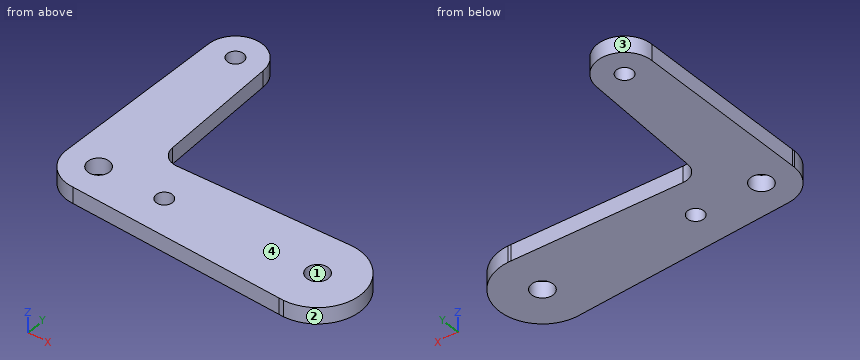
```python
from build123d import *

# Parameters (mm, degrees)
BOSS_EXTRUDE1_DEPTH = 4.7752
FILLET1_R           = 4.7752
SKETCH2_R           = 3.175
SKETCH2_R_2         = 2.3876
CUT_EXTRUDE1_DEPTH  = 4.7752


with BuildPart() as part:
    # Sketch1 → Boss-Extrude1 (new body)
    with BuildSketch(Plane.XY):
        with BuildLine():
            ThreePointArc((7.9502, 50.8), (0, 58.7502), (-7.9502, 50.8))
            Line((-7.9502, 50.8), (-9.506710526, 0.589983026))
            Line((-9.506710526, 0.589983026), (-9.525, 0))
            ThreePointArc((-9.525, 0), (-6.735192091, -6.735192091), (0, -9.525))
            Line((0, -9.525), (62.233167082, -12.636658354))
            Line((62.233167082, -12.636658354), (63.5, -12.7))
            ThreePointArc((63.5, -12.7), (76.2, 0), (63.5, 12.7))
            Line((63.5, 12.7), (62.713355965, 12.675614035))
            Line((62.713355965, 12.675614035), (9.183498158, 11.016188443))
            Line((9.183498158, 11.016188443), (7.9502, 50.8))
        make_face()
        with BuildLine():
            ThreePointArc((9.506710526, 0.589983026), (9.520426534, 0.295133223), (9.525, 0))
            Line((9.525, 0), (9.506710526, 0.589983026))
        make_face(mode=Mode.SUBTRACT)
    extrude(amount=BOSS_EXTRUDE1_DEPTH)

    # Fillet1
    fillet1_edges = [part.edges().sort_by_distance(p)[0] for p in [
        (9.183498158, 11.016188443, 2.3876),
    ]]
    fillet(fillet1_edges, radius=FILLET1_R)

    # Sketch2 → Cut-Extrude1 (cut)
    with BuildSketch(Plane.XY.offset(4.7752)):
        Circle(SKETCH2_R)
        with Locations((0, 50.8)):
            Circle(SKETCH2_R_2)
        with Locations((19.05, 0)):
            Circle(SKETCH2_R_2)
        with Locations((63.5, 0)):
            Circle(SKETCH2_R)
    extrude(amount=-CUT_EXTRUDE1_DEPTH, mode=Mode.SUBTRACT)


solid = part.part
```
Work out the finished part from the listing and answer in its coordinate system (mm). Face numbers are marked on the shaded views. Give positions to 0.01 mm unless a question says otherwise; leave off trailing zeros. Loops run counter-clockwise (first coordinate to the right, second up) from the corner with the lowest first, then second, coordinate; pieces in that order, holes last. Notation, with made-up numbers: (65.25, 45.5) -> (82.25, 45.5) arc R37 cw to (82.25, 84.5) -> close; hole circle Ø5 at (17, -14). An arc over 180 degrees is marked (long way). One line per question, with ' | ' between items. Start each with the question number.
1) Section C-C, the plane y = 18 is taken. Determine the outline of the cut face in (x, z).
2) Section B-B, the plane x = 19.5 is taken. Determine the outline of the cut face in (y, z).
3) Determine the mould class of the marked faces 1, 2, 3 and 4 for opening direction X: +X half, -X half, draft (parallel to the pull), parting line (faces both ways), or undercut.
4) Section A-A, the plane z = 3.3 is taken. Determine the outline of the cut face in (x, y) (3 decimals).
5) This flat-tipped pin is pushed along its axis until it touches: pin 1 (1.5 mm diameter, centred on y = 31, z = 3.5, fed in from -X). Where does it stop, or does it pass through?
6) Straight lines are drawn through the part: L1, parallel to Y at x = 0, z = 2.9 (3 decimals); L2, parallel to Y at x = 63.5, z = 1.85 (3 decimals); L3, parallel to Y at x = 19.5, z = 0.3. For each, find the intervals that lie inside material, in ascending order.
7) Section D-D, the plane x = 55.5 is taken. Determine the outline of the cut face in (y, z), then the cut area to 3 significant figures.
Resolved:
1) outline: (-8.97, 0) -> (8.97, 0) -> (8.97, 4.78) -> (-8.97, 4.78) -> close
2) outline: (-10.5, 0) -> (-2.34, 0) -> (-2.34, 4.78) -> (-10.5, 4.78) -> close; (2.34, 0) -> (11.34, 0) -> (11.34, 4.78) -> (2.34, 4.78) -> close
3) face 1: undercut | face 2: +X half | face 3: parting line | face 4: draft
4) outline: (-9.525, 0) arc R9.525 ccw to (0, -9.525) -> (63.5, -12.7) arc R12.7 ccw to (63.5, 12.7) -> (13.956, 11.164) arc R4.775 cw to (9.036, 15.789) -> (7.95, 50.8) arc R7.95 ccw to (-7.95, 50.8) -> close; hole circle Ø6.35 at (0, 0); hole circle Ø4.775 at (0, 50.8); hole (9.507, 0.59) -> (9.525, 0) arc R9.525 ccw to start; hole circle Ø4.775 at (19.05, 0); hole circle Ø6.35 at (63.5, 0)
5) pin 1: x = -8.59
6) L1: -9.525 to -3.175, 3.175 to 48.412, 53.188 to 58.75 | L2: -12.7 to -3.175, 3.175 to 12.7 | L3: -10.5 to -2.34, 2.34 to 11.34
7) outline: (-12.3, 0) -> (12.45, 0) -> (12.45, 4.78) -> (-12.3, 4.78) -> close | area: 118 mm2
